```python
from build123d import *

# Parameters (mm, degrees)
SKETCH_1_R      = 2.25
EXTRUDE_1_DEPTH = 4.5


with BuildPart() as part:
    # 草图1 → 凸台-拉伸1 (new body)
    with BuildSketch(Plane(origin=(0, 0, 0), x_dir=(0, 0, -1), z_dir=(1, 0, 0))):
        with BuildLine():
            Line((0, 0), (20, 0))
            Line((20, 0), (20, 28))
            ThreePointArc((20, 28), (10, 38), (0, 28))
            Line((0, 28), (0, 0))
        make_face()
        with Locations((10, 28)):
            Circle(SKETCH_1_R, mode=Mode.SUBTRACT)
        with Locations((10, 7)):
            Circle(SKETCH_1_R, mode=Mode.SUBTRACT)
    extrude(amount=EXTRUDE_1_DEPTH)


solid = part.part
```
The model under review builds one solid part; all positions refer to its coordinate system, in mm. Round coordinates to 2 decimals unless told otherwise and drop trailing zeros. Loops run counter-clockwise (first coordinate to the right, second up) from the corner with the lowest first, then second, coordinate; pieces in that order, holes last.
Item 1: Take a section at C-C (x = 1.7). Write out the cut boundary in (y, z), then the cut area to 3 significant figures.
Determined:
outline: (0, -20) - (28, -20) arc R10 ccw to (28, 0) - (0, 0) - close; hole circle Ø4.5 at (7, -10); hole circle Ø4.5 at (28, -10)
area: 685 mm2
Item 2: Take a section at D-D (z = -4). Write out the cut boundary in (x, y), then the cut area to 3 significant figures.
Determined:
outline: (0, 0) - (4.5, 0) - (4.5, 36) - (0, 36) - close
area: 162 mm2
Item 3: Mouldability with a two-part tool opening along Y and no side actions: class faces 1 (the face through (2.22, 8.52, -8.34)), 2 (the face through (2, 0, -10)), 3 (the face through (2.218, 25.804, -9.512)), 4 (the face through (2, 38, -10)) as released by +Y, released by -Y, zero draft, split by the parting line, or undercut.
Determined:
face 1: undercut
face 2: released by -Y
face 3: undercut
face 4: released by +Y
Item 4: For line 1 (Y direction, x = 2, z = -10); line 2 (Z direction, x = 2.35, y = 5.5); line 3 (Z direction, x = 2.75, y = 34), list the stretches that pass through material, from the lowest coordinate up.
Determined:
line 1: y = 0 to 4.75, 9.25 to 25.75, 30.25 to 38
line 2: z = -20 to -11.68, -8.32 to 0
line 3: z = -18 to -2
Item 5: Take a section at A-A (z = -10). Write out the cut boundary in (x, y).
Determined:
outline: (0, 0) - (4.5, 0) - (4.5, 4.75) - (0, 4.75) - close; (0, 9.25) - (4.5, 9.25) - (4.5, 25.75) - (0, 25.75) - close; (0, 30.25) - (4.5, 30.25) - (4.5, 38) - (0, 38) - close
Item 6: Take a section at B-B (y = 7). Write out the cut boundary in (x, z).
Determined:
outline: (0, -20) - (4.5, -20) - (4.5, -12.25) - (0, -12.25) - close; (0, -7.75) - (4.5, -7.75) - (4.5, 0) - (0, 0) - close
